Study the drawing (mm; zero at the part's minimum x, y, z) and answer. A direction names the side the tool comes from. Coordinates: 2 decimals unless noted, no trailing zeros. Order: outer loops, then holes, each group sorted by start corner. A loop starts at its lowest first (then second) coordinate and runs counter-clockwise, first axis right, second up.
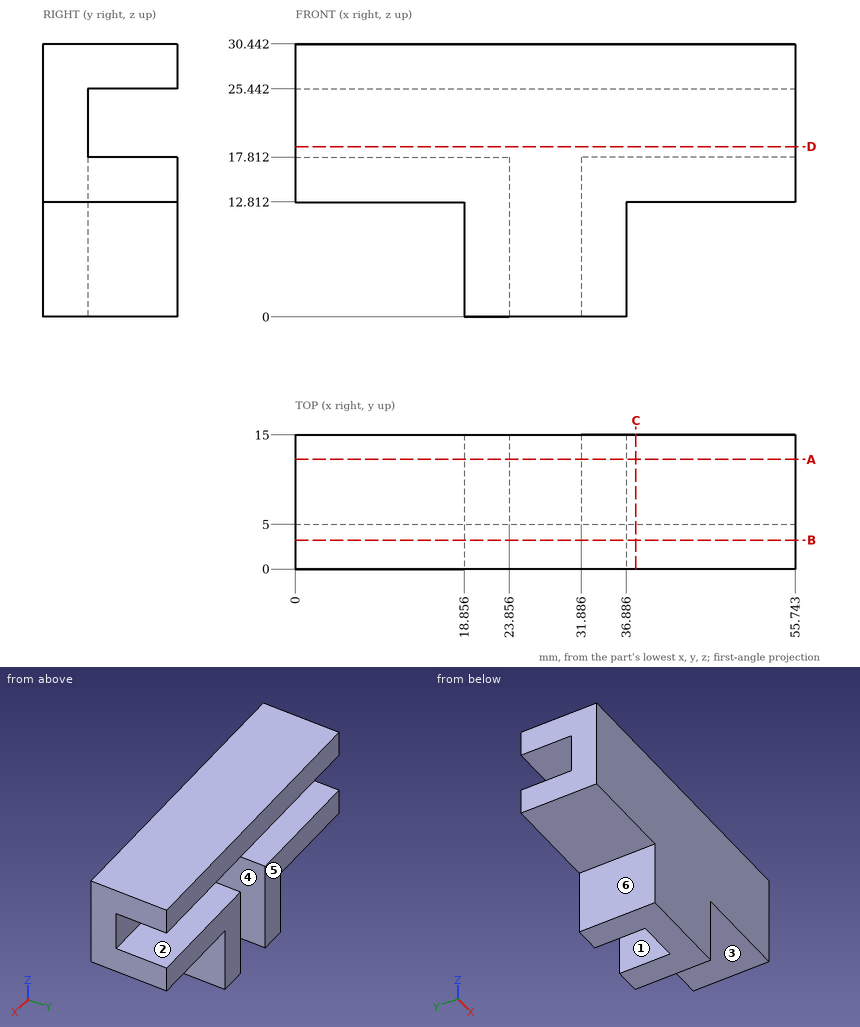
1) A cutting plane is placed at C-C, the plane x = 38. Determine the outline of the cut face in (y, z), and give its area (3 significant figures).
A:
outline: (0, 12.81) - (15, 12.81) - (15, 17.81) - (5, 17.81) - (5, 25.44) - (15, 25.44) - (15, 30.44) - (0, 30.44) - close
area: 188 mm2
2) A cutting plane is placed at A-A, the plane y = 12.25. Determine the outline of the cut face in (x, z).
A:
outline: (0, 12.81) - (18.86, 12.81) - (18.86, 0) - (23.86, 0) - (23.86, 17.81) - (0, 17.81) - close; (0, 25.44) - (55.74, 25.44) - (55.74, 30.44) - (0, 30.44) - close; (31.89, 0) - (36.89, 0) - (36.89, 12.81) - (55.74, 12.81) - (55.74, 17.81) - (31.89, 17.81) - close
3) A cutting plane is placed at B-B, the plane y = 3.25. Determine the outline of the cut face in (x, z), and give its area (3 significant figures).
A:
outline: (0, 12.81) - (18.86, 12.81) - (18.86, 0) - (36.89, 0) - (36.89, 12.81) - (55.74, 12.81) - (55.74, 30.44) - (0, 30.44) - close
area: 1,210 mm2
4) Straight lines are drawn through the part: line 1 (X direction, y = 6.5, z = 6); line 2 (Z direction, x = 18, y = 10); line 3 (X direction, y = 12.5, z = 14). For each, find the intervals that lie inside material, in ascending order.
A:
line 1: x = 18.86 to 23.86, 31.89 to 36.89
line 2: z = 12.81 to 17.81, 25.44 to 30.44
line 3: x = 0 to 23.86, 31.89 to 55.74
5) Determine the mould class of the marked faces 4, 5 and 6 for opening direction X: pulls with the +X half, pulls with the -X half, needs draft (parallel to the pull), parting line crosses it, or undercut.
A:
face 4: undercut
face 5: needs draft
face 6: pulls with the -X half
6) Flat-ended cylindrical pins translate along their axes: pin 1 Ø8 at (y, z) = (12, 8) entering from -X; pin 2 Ø6.5 at (y, z) = (8.5, 7) entering from +X; pin 3 Ø5 at (x, y) = (27.5, 8.5) entering from -Z. Find the tip coordinate at first contact, or state that the pin passes through.
A:
pin 1: stops at x = 18.86
pin 2: stops at x = 36.89
pin 3: stops at z = 25.44
7) Which of the six approach directions +Z, -Z, +X, -X, +Y, -Y give full straight-line access (tool end or side, diameter ignored) to the marked faces 1, 2 and 3?
A:
face 1: -Z, +Y
face 2: +X, -X, +Y
face 3: -Z, +X, +Y, -Y
8) A cutting plane is placed at D-D, the plane z = 19. Determine the outline of the cut face in (x, y).
A:
outline: (0, 0) - (55.74, 0) - (55.74, 5) - (0, 5) - close
